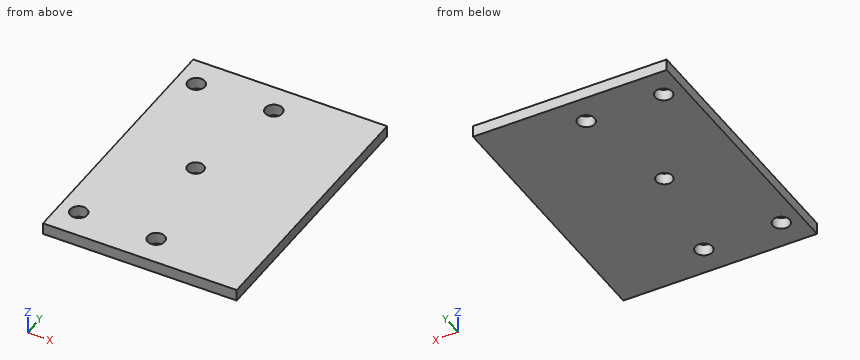
```python
from build123d import *

# Parameters (mm, degrees)
SKETCH_1_W          = 40
SKETCH_1_H          = 29
EXTRUDE_1_DEPTH     = 3
SKETCH_3_W          = 40
SKETCH_3_H          = 3
EXTRUDE_2_DEPTH     = 3
SKETCH_4_W          = 40
SKETCH_4_H          = 3
EXTRUDE_3_DEPTH     = 3
SKETCH_5_W          = 40
SKETCH_5_H          = 3
EXTRUDE_4_DEPTH     = 7
SKETCH_6_W          = 40
SKETCH_6_H          = 3
EXTRUDE_5_DEPTH     = 7
SKETCH_7_W          = 40
SKETCH_7_H          = 3
EXTRUDE_6_DEPTH     = 10
SKETCH_8_W          = 40
SKETCH_8_H          = 3
EXTRUDE_7_DEPTH     = 10
SKETCH_12_W         = 3
SKETCH_12_H         = 69
EXTRUDE_9_DEPTH     = 30
SKETCH_15_R         = 2.1
CUT_EXTRUDE_4_DEPTH = 10
SKETCH_16_W         = 3
SKETCH_16_H         = 69
CUT_EXTRUDE_5_DEPTH = 20
SKETCH_17_R         = 2.2
CUT_EXTRUDE_6_DEPTH = 10


with BuildPart() as part:
    # ｽｹｯﾁ1 → ﾎﾞｽ - 押し出し1 (new body)
    with BuildSketch(Plane.XY):
        Rectangle(SKETCH_1_W, SKETCH_1_H)
    extrude(amount=EXTRUDE_1_DEPTH)

    # ｽｹｯﾁ3 → ﾎﾞｽ - 押し出し2 (add)
    with BuildSketch(Plane(origin=(0, -14.5, 0), x_dir=(-1, 0, 0), z_dir=(0, -1, 0))):
        with Locations((0, -1.5)):
            Rectangle(SKETCH_3_W, SKETCH_3_H)
    extrude(amount=EXTRUDE_2_DEPTH)

    # ｽｹｯﾁ4 → ﾎﾞｽ - 押し出し3 (add)
    with BuildSketch(Plane(origin=(0, 14.5, 0), x_dir=(1, 0, 0), z_dir=(0, 1, 0))):
        with Locations((0, -1.5)):
            Rectangle(SKETCH_4_W, SKETCH_4_H)
    extrude(amount=EXTRUDE_3_DEPTH)

    # ｽｹｯﾁ5 → ﾎﾞｽ - 押し出し4 (add)
    with BuildSketch(Plane.XZ.offset(17.5)):
        with Locations((0, 1.5)):
            Rectangle(SKETCH_5_W, SKETCH_5_H)
    extrude(amount=EXTRUDE_4_DEPTH)

    # ｽｹｯﾁ6 → ﾎﾞｽ - 押し出し5 (add)
    with BuildSketch(Plane(origin=(0, 17.5, 0), x_dir=(1, 0, 0), z_dir=(0, 1, 0))):
        with Locations((0, -1.5)):
            Rectangle(SKETCH_6_W, SKETCH_6_H)
    extrude(amount=EXTRUDE_5_DEPTH)

    # ｽｹｯﾁ7 → ﾎﾞｽ - 押し出し6 (add)
    with BuildSketch(Plane(origin=(0, 24.5, 0), x_dir=(1, 0, 0), z_dir=(0, 1, 0))):
        with Locations((0, -1.5)):
            Rectangle(SKETCH_7_W, SKETCH_7_H)
    extrude(amount=EXTRUDE_6_DEPTH)

    # ｽｹｯﾁ8 → ﾎﾞｽ - 押し出し7 (add)
    with BuildSketch(Plane.XZ.offset(24.5)):
        with Locations((0, 1.5)):
            Rectangle(SKETCH_8_W, SKETCH_8_H)
    extrude(amount=EXTRUDE_7_DEPTH)

    # ｽｹｯﾁ12 → ﾎﾞｽ - 押し出し9 (add)
    with BuildSketch(Plane.ZY.offset(20)):
        with Locations((1.5, 0)):
            Rectangle(SKETCH_12_W, SKETCH_12_H)
    extrude(amount=EXTRUDE_9_DEPTH)

    # ｽｹｯﾁ15 → ｶｯﾄ - 押し出し4 (cut)
    with BuildSketch(Plane.XY.offset(3)):
        with Locations((-10, 0)):
            Circle(SKETCH_15_R)
    extrude(amount=-CUT_EXTRUDE_4_DEPTH, mode=Mode.SUBTRACT)

    # ｽｹｯﾁ16 → ｶｯﾄ - 押し出し5 (cut)
    with BuildSketch(Plane.ZY.offset(50)):
        with Locations((1.5, 0)):
            Rectangle(SKETCH_16_W, SKETCH_16_H)
    extrude(amount=-CUT_EXTRUDE_5_DEPTH, mode=Mode.SUBTRACT)

    # ｽｹｯﾁ17 → ｶｯﾄ - 押し出し6 (cut)
    with BuildSketch(Plane(origin=(0, 0, 0), x_dir=(-1, 0, 0), z_dir=(0, 0, -1))):
        with Locations((5, 27)):
            Circle(SKETCH_17_R)
        with Locations((25, 27)):
            Circle(SKETCH_17_R)
        with Locations((5, -27)):
            Circle(SKETCH_17_R)
        with Locations((25, -27)):
            Circle(SKETCH_17_R)
    extrude(amount=-CUT_EXTRUDE_6_DEPTH, mode=Mode.SUBTRACT)


solid = part.part
```
Check sheet for the modelled part. Datum: model origin and axes. Units: mm. Give positions to 0.01 mm unless a question says otherwise; leave off trailing zeros. Write each loop counter-clockwise with the first axis right and the second up, starting at its lowest first coordinate (ties: lowest second). Pieces come first, ordered by that corner, then holes. Notation, with made-up numbers: (14.5, 77) - (56.5, 77) arc R23 cw to (56.5, 105) - close; hole circle Ø8 at (40, 69.25). An arc over 180 degrees is marked (long way). Answer as a JSON object with one key per item and string values. Group by question number.
1) Depth check by flat-ended pin: P1, Ø7, axis at x = -25, y = -27, coming from the +Z side. Enter the tip coordinate at first touch or a pass-through.
2) Thickness scan on probe 1 along Y at (x, z) = (-5, 2.35); probe 2 along Y at (x, z) = (-10, 1.7); probe 3 along Y at (x, z) = (-23, 2.5). Record the ranges inside material, lowest first. Write a range as from..to.
3) Sectioned sample at C-C (x = -25). Record the cut outline in (y, z).
4) Sectioned sample at D-D (z = 2.55). Record the cut outline in (x, y), then the cut area to 3 significant figures.
5) Sectioned sample at B-B (y = 0). Record the cut outline in (x, z), then the cut area to 3 significant figures.
6) Sectioned sample at A-A (x = -10). Record the cut outline in (y, z), then the cut area to 3 significant figures.
Geometry results:
{
 "1": {"P1": "stops at z = 3"},
 "2": {"probe 1": "y = -34.5..-29.2, -24.8..24.8, 29.2..34.5", "probe 2": "y = -34.5..-2.1, 2.1..34.5", "probe 3": "y = -34.5..-27.92, -26.08..26.08, 27.92..34.5"},
 "3": {"outline": "(-34.5, 0) - (-29.2, 0) - (-29.2, 3) - (-34.5, 3) - close; (-24.8, 0) - (24.8, 0) - (24.8, 3) - (-24.8, 3) - close; (29.2, 0) - (34.5, 0) - (34.5, 3) - (29.2, 3) - close"},
 "4": {"outline": "(-30, -34.5) - (20, -34.5) - (20, 34.5) - (-30, 34.5) - close; hole circle Ø4.4 at (-25, -27); hole circle Ø4.4 at (-25, 27); hole circle Ø4.2 at (-10, 0); hole circle Ø4.4 at (-5, -27); hole circle Ø4.4 at (-5, 27)", "area": "3,380 mm^2"},
 "5": {"outline": "(-30, 0) - (-12.1, 0) - (-12.1, 3) - (-30, 3) - close; (-7.9, 0) - (20, 0) - (20, 3) - (-7.9, 3) - close", "area": "137 mm^2"},
 "6": {"outline": "(-34.5, 0) - (-2.1, 0) - (-2.1, 3) - (-34.5, 3) - close; (2.1, 0) - (34.5, 0) - (34.5, 3) - (2.1, 3) - close", "area": "194 mm^2"}
}
